Study the drawing (mm; zero at the part's minimum x, y, z) and answer. Coordinates: 2 decimals unless noted, no trailing zeros. Order: outer loops, then holes, each group sorted by start corner. A loop starts at its lowest first (then second) coordinate and runs counter-clockwise, first axis right, second up. Notation, with made-up numbers: M 17.25,85 L 43.25,85 A21 cw 43.25,101 Z; hole C 74,58 d4. An arc over 180 degrees is marked long. One line per item, written item: value. Start each with the question number.
Q1. Straight lines are drawn through the part: line 1 along X through (y, z) = (28, 3); line 2 along X through (y, z) = (14, 4.75); line 3 along Y through (x, z) = (17, 4). For each, find the intervals that lie inside material, in ascending order. Write a range as [from, to].
Q2. The part is cut by section A-A on y = 21.25. Give the vertices of the cut face in (x, z).
Q3. The part is cut by section D-D on x = 27. Give the vertices of the cut face in (y, z).
Q4. The part is cut by section C-C on x = 76. Give the vertices of the cut face in (y, z).
Q5. Determine the mould class of the marked faces 1, 2 and 3 for opening direction Y: pulls with the +Y half, pulls with the -Y half, needs draft (parallel to the pull), parting line crosses it, or undercut.
Q6. The part is cut by section B-B on z = 6. Give the vertices of the cut face in (x, y), then the cut area to 3 significant figures.
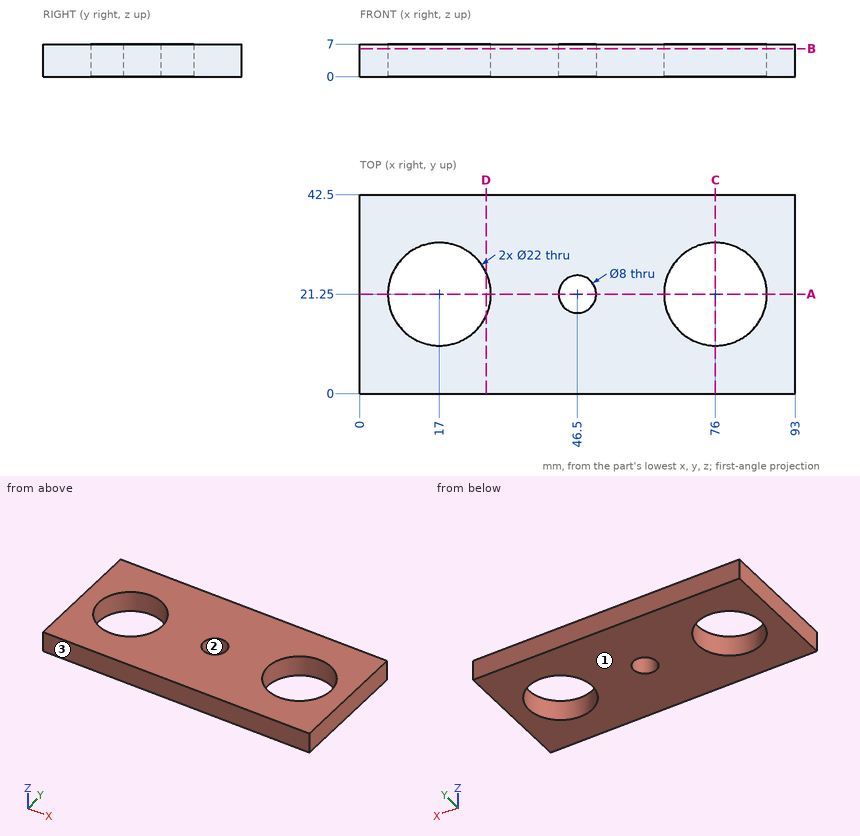
Output:
1. line 1: x = [0, 8.31], [25.69, 67.31], [84.69, 93]
1. line 2: x = [0, 8.73], [25.27, 67.73], [84.27, 93]
1. line 3: y = [0, 10.25], [32.25, 42.5]
2. outline: M 0,0 L 6,0 L 6,7 L 0,7 Z; M 28,0 L 42.5,0 L 42.5,7 L 28,7 Z; M 50.5,0 L 65,0 L 65,7 L 50.5,7 Z; M 87,0 L 93,0 L 93,7 L 87,7 Z
3. outline: M 0,0 L 16.67,0 L 16.67,7 L 0,7 Z; M 25.83,0 L 42.5,0 L 42.5,7 L 25.83,7 Z
4. outline: M 0,0 L 10.25,0 L 10.25,7 L 0,7 Z; M 32.25,0 L 42.5,0 L 42.5,7 L 32.25,7 Z
5. face 1: needs draft
5. face 2: undercut
5. face 3: pulls with the -Y half
6. outline: M 0,0 L 93,0 L 93,42.5 L 0,42.5 Z; hole C 17,21.25 d22; hole C 46.5,21.25 d8; hole C 76,21.25 d22
6. area: 3,140 mm^2
